Here's the drawing with two shaded views (mm, measured from the low corner). I have some questions. A direction names the side the tool comes from. Give positions to 0.01 mm unless a question says otherwise; leave off trailing zeros. Loops run counter-clockwise (first coordinate to the right, second up) from the corner with the lowest first, then second, coordinate; pieces in that order, holes last. Notation, with made-up numbers: (17, -35) - (35, -35) arc R20 ccw to (35, -14) - close; hole circle Ø8 at (-3.5, -32.75). An arc over 180 degrees is marked (long way). Use one line per item in the form item = value.
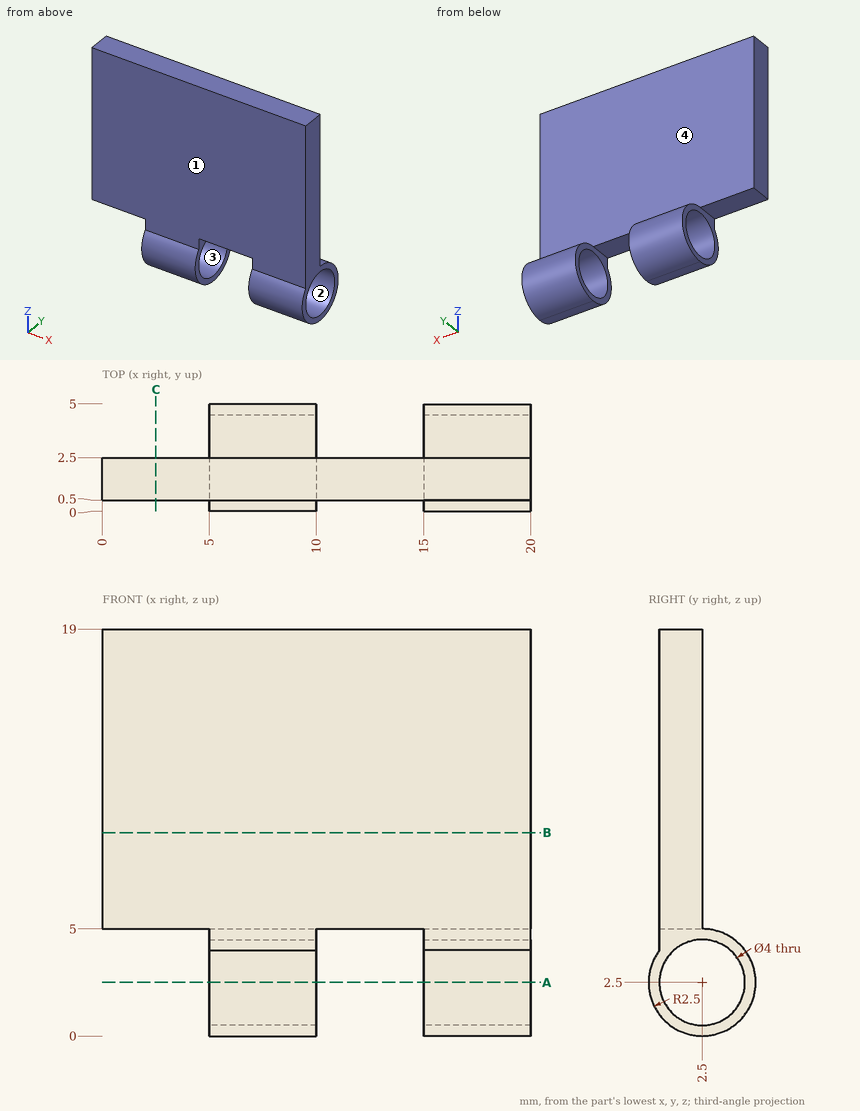
(1) Thinking about a two-plate mould opening in Z: for the marked faces 1 and 2, which applies, pulls with the +Z half, pulls with the -Z half, needs draft (parallel to the pull), parting line crosses it, or undercut?
Geometry says:
face_1 = needs draft
face_2 = undercut
(2) For P1, Ø1, axis at y = 2.5, z = 15, coming from the -X side; P2, Ø11, axis at x = 11.5, z = 10, coming from the +Y side; P3, Ø1.5, axis at y = 1.5, z = 3.5, coming from the -X side; P4, Ø0.6, axis at x = 11.5, y = 1.5, coming from the -Z side, each with a flat end and sliding along its axis, tell me the tip position at first contact or that it passes through.
Geometry says:
P1 = 0
P2 = 3.67
P3 = 5
P4 = 5
(3) If we section it at C-C (x = 2.5): List the corners of the cut face in (y, z) for me, plus the area to 3 significant figures.
Geometry says:
outline = (0.5, 5) - (2.5, 5) - (2.5, 19) - (0.5, 19) - close
area = 28.0 mm²
(4) If we section it at B-B (z = 9.5): List the corners of the cut face in (x, y) for me.
Geometry says:
outline = (0, 0.5) - (20, 0.5) - (20, 2.5) - (0, 2.5) - close
(5) For the marked faces 3 and 4, which set-ups out of +Z, -Z, +X, -X, +Y, -Y let a thin tool reach every point of the face, with its end or its side?
Geometry says:
face_3 = +X, -X
face_4 = +Z, +X, -X, +Y
(6) If we section it at A-A (z = 2.5): List the corners of the cut face in (x, y) for me.
Geometry says:
outline = (5, 0) - (10, 0) - (10, 0.5) - (5, 0.5) - close; (5, 4.5) - (10, 4.5) - (10, 5) - (5, 5) - close; (15, 0) - (20, 0) - (20, 0.5) - (15, 0.5) - close; (15, 4.5) - (20, 4.5) - (20, 5) - (15, 5) - close
(7) If I drill on probe 1 along X at (y, z) = (3.6, 4.25); probe 2 along Y at (x, z) = (17.1, 2.5); probe 3 along Z at (x, y) = (15.5, 2.45), over which ranges is the centre line in solid material (lowest first)?
Geometry says:
probe_1 = 5 to 10, 15 to 20
probe_2 = 0 to 0.5, 4.5 to 5
probe_3 = 0 to 0.5, 4.5 to 19
